Geometry: final body of the model. Coordinates: model frame, mm. A direction names the side the tool comes from. Coordinates: 2 decimals unless noted, no trailing zeros. Order: outer loops, then holes, each group sorted by start corner. A loop starts at its lowest first (then second) coordinate and runs counter-clockwise, first axis right, second up. Notation, with made-up numbers: M -4.5,-23.75 L 4.5,-23.75 A6 cw 4.5,-17.75 Z; hole C 44,65.25 d6. An arc over 180 degrees is marked long. Use CSV: the item, a comma, the result in double quotes. Start each with the question number.
1. Pull-direction query (X, two-part tool) for faces 4 (the flat face through (12, 2, -5)), 5 (the flat face through (-5.5, 3, -21)), 6 (the flat face through (-7.5, 11, -3)), 7 (the flat face through (7.5, 10, -3)); classes: pulls with the +X half, pulls with the -X half, needs draft (parallel to the pull), parting line crosses it, or undercut.
2. Section query C-C on z = -4.5. Return the cut outline in (x, y), and give its area (3 significant figures).
3. Section query A-A on y = -2.5. Return the cut outline in (x, z), and give its area (3 significant figures).
4. Section query B-B on x = -1.75. Return the cut outline in (y, z), and give its area (3 significant figures).
5. Material intervals for line 1 (X direction, y = 5.5, z = -17); line 2 (X direction, y = 13.5, z = -3.5); line 3 (Y direction, x = 7, z = -1), sorted ascending.
6. Section query D-D on z = -23. Return the cut outline in (x, y), and give its area (3 significant figures).
7. First-contact query: P1, Ø12, axis at x = -2, z = -21.5, coming from the -Y side; P2, Ø2, axis at x = 4, z = -13.5, coming from the +Y side; P3, Ø0.8, axis at x = 4.5, y = 6.5, coming from the -Z side; P4, Ø8, axis at x = 6.5, y = 5.5, coming from the +Z side. Flat tips, straight axial feed; report the tip coordinate or a pass-through.
8. Set-up query: faces 1 (the flat face through (5.5, 3, -21)), 2 (the flat face through (3.466, 6.5, -10.4)), 3 (the flat face through (0, 1.5, -21)). Return all of +Z, -Z, +X, -X, +Y, -Y with unobstructed straight access to the full face (end or side cutting, diameter ignored); none if empty.
from build123d import *

# Parameters (mm, degrees)
F1_DEPTH = 6
F3_DEPTH = 6
F5_DEPTH = 30
F6_W     = 2
F6_H     = 1
F7_DEPTH = 21


with BuildPart() as f1:
    # F0 (on Top) → F1 (new body)
    with BuildSketch(Plane.XY):
        with BuildLine():
            ThreePointArc((12, 16), (11.1213203436, 18.1213203436), (9, 19))
            Line((9, 19), (-9, 19))
            ThreePointArc((-9, 19), (-11.1213203436, 18.1213203436), (-12, 16))
            Line((-12, 16), (-12, -16))
            ThreePointArc((-12, -16), (-11.1213203436, -18.1213203436), (-9, -19))
            Line((-9, -19), (9, -19))
            ThreePointArc((9, -19), (11.1213203436, -18.1213203436), (12, -16))
            Line((12, -16), (12, 16))
        make_face()
    extrude(amount=-F1_DEPTH)

    # F2 (on face) → F3 (cut, through all)
    with BuildSketch(Plane.XY):
        with BuildLine():
            ThreePointArc((7.5, 15), (6.6213203436, 17.1213203436), (4.5, 18))
            Line((4.5, 18), (-4.5, 18))
            ThreePointArc((-4.5, 18), (-6.6213203436, 17.1213203436), (-7.5, 15))
            Line((-7.5, 15), (-7.5, 6))
            Line((-7.5, 6), (7.5, 6))
            Line((7.5, 6), (7.5, 15))
        make_face()
        with BuildLine():
            Line((7.5, -14.5), (7.5, -0.5))
            Line((7.5, -0.5), (-7.5, -0.5))
            Line((-7.5, -0.5), (-7.5, -14.5))
            ThreePointArc((-7.5, -14.5), (-6.6213203436, -16.6213203436), (-4.5, -17.5))
            Line((-4.5, -17.5), (4.5, -17.5))
            ThreePointArc((4.5, -17.5), (6.6213203436, -16.6213203436), (7.5, -14.5))
        make_face()
    extrude(amount=-F3_DEPTH, mode=Mode.SUBTRACT)

    # F4 (on face) → F5 (join)
    with BuildSketch(Plane(origin=(0, 0, -6), x_dir=(1, 0, 0), z_dir=(0, 0, -1))):
        Polygon((-3.5, -2.5), (3.5, -2.5), (3.5, -6), (7.5, -6), (12, -6), (12, -4), (5.5, -4), (5.5, -1.5), (-5.5, -1.5), (-5.5, -4), (-12, -4), (-12, -6), (-7.5, -6), (-3.5, -6), align=None)
    extrude(amount=F5_DEPTH)

    # F6 (on face) → F7 (join)
    with BuildSketch(Plane.XY):
        with Locations((-4.5, 6.5)):
            Rectangle(F6_W, F6_H)
        with Locations((4.4662822727, 6.5)):
            Rectangle(F6_W, F6_H)
    extrude(amount=-F7_DEPTH)


solid = f1.part
Results list:
1,face 4,"pulls with the +X half"
1,face 5,"pulls with the -X half"
1,face 6,"undercut"
1,face 7,"undercut"
2,outline,"M -12,-16 A3 ccw -9,-19 L 9,-19 A3 ccw 12,-16 L 12,16 A3 ccw 9,19 L -9,19 A3 ccw -12,16 Z; hole M -7.5,-14.5 A3 ccw -4.5,-17.5 L 4.5,-17.5 A3 ccw 7.5,-14.5 L 7.5,-0.5 L -7.5,-0.5 Z; hole M -7.5,6 L -5.5,6 L -5.5,7 L -3.5,7 L -3.5,6 L 3.47,6 L 3.47,7 L 5.47,7 L 5.47,6 L 7.5,6 L 7.5,15 A3 ccw 4.5,18 L -4.5,18 A3 ccw -7.5,15 Z"
2,area,"481 mm²"
3,outline,"M -12,-6 L -7.5,-6 L -7.5,0 L -12,0 Z; M 7.5,-6 L 12,-6 L 12,0 L 7.5,0 Z"
3,area,"54.0 mm²"
4,outline,"M -19,-6 L -17.5,-6 L -17.5,0 L -19,0 Z; M -0.5,-6 L 1.5,-6 L 1.5,-36 L 2.5,-36 L 2.5,-6 L 6,-6 L 6,0 L -0.5,0 Z; M 18,-6 L 19,-6 L 19,0 L 18,0 Z"
4,area,"84.0 mm²"
5,line 1,"x = -12 to -3.5, 3.5 to 12"
5,line 2,"x = -12 to -7.5, 7.5 to 12"
5,line 3,"y = -19 to -16.16, -0.5 to 6, 16.66 to 19"
6,outline,"M -12,4 L -5.5,4 L -5.5,1.5 L 5.5,1.5 L 5.5,4 L 12,4 L 12,6 L 3.5,6 L 3.5,2.5 L -3.5,2.5 L -3.5,6 L -12,6 Z"
6,area,"51.0 mm²"
7,P1,"stops at y = 1.5"
7,P2,"stops at y = 7"
7,P3,"stops at z = -21"
7,P4,"stops at z = 0"
8,face 1,"-Z, +X, -Y"
8,face 2,"+Z, -Z"
8,face 3,"-Z, +X, -X, -Y"
